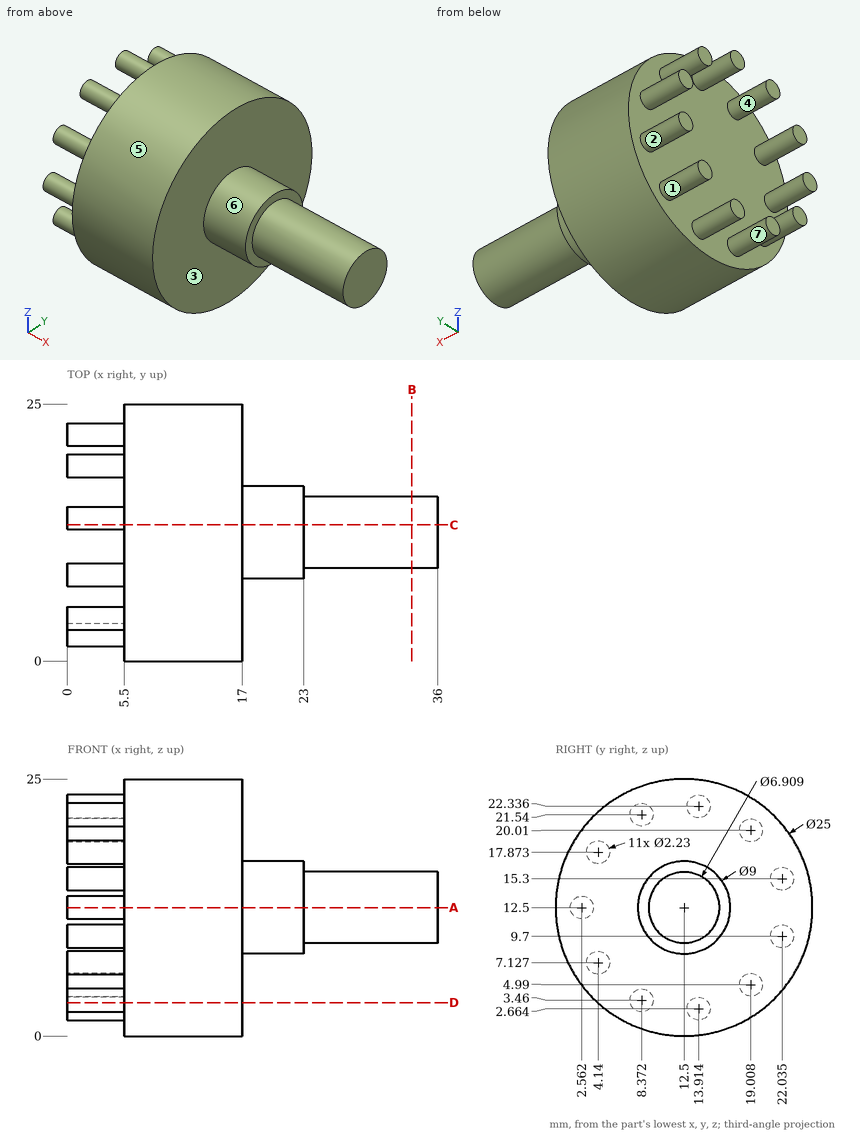
Here's the drawing with two shaded views (mm, measured from the low corner). I have some questions. A direction names the side the tool comes from. Give positions to 0.01 mm unless a question says otherwise; leave off trailing zeros. Write each loop counter-clockwise with the first axis right and the second up, starting at its lowest first coordinate (ties: lowest second). Pieces come first, ordered by that corner, then holes. Notation, with made-up numbers: (66.25, -36) -> (109.25, -36) arc R25 ccw to (109.25, -17) -> close; hole circle Ø8 at (83, 0.5). An arc over 180 degrees is marked (long way). Use one line per item in the form item = value. Start each with the question number.
1. Imagine slicing it at C-C on y = 13.25. List the corners of the cut face in (x, z) for me.
2. Imagine slicing it at A-A on z = 12.5. List the corners of the cut face in (x, y) for me (1 decimal).
3. On a 3-axis mill with a long thin cutter (end or side, diameter ignored), from which of +Z, -Z, +X, -X, +Y, -Y can I reach the whole of each face in a straight line? I mean the marked faces 5, 6 and 7. Say none if no direction works.
4. Will these pins go through, and if not, where does the flat tip stop? pin 1 Ø12 at (x, z) = (11.5, 19) entering from -Y; pin 2 Ø8 at (x, z) = (4.5, 3.5) entering from -Y; pin 3 Ø2 at (x, y) = (11.5, 2.5) entering from -Z (1 decimal).
5. If I drill on L1, parallel to X at y = 16.5, z = 21.25; L2, parallel to Z at x = 3, y = 2.5; L3, parallel to X at y = 8.5, z = 2.75, over which ranges is the centre line in solid material (lowest first)?
6. Imagine slicing it at D-D on z = 3.25. List the corners of the cut face in (x, y) for me.
7. Thinking about a two-plate mould opening in Y: for the marked faces 1, 2, 3 and 4, which applies, +Y half, -Y half, draft (parallel to the pull), parting line (faces both ways), or undercut?
8. Imagine slicing it at B-B on x = 33.5. List the corners of the cut face in (y, z) for me (1 decimal), plus the area to 3 significant figures.
Entries:
q1.outline = (0, 1.77) -> (5.5, 1.77) -> (5.5, 0.02) -> (17, 0.02) -> (17, 8.06) -> (23, 8.06) -> (23, 9.13) -> (36, 9.13) -> (36, 15.87) -> (23, 15.87) -> (23, 16.94) -> (17, 16.94) -> (17, 24.98) -> (5.5, 24.98) -> (5.5, 23.23) -> (0, 23.23) -> (0, 21.44) -> (5.5, 21.44) -> (5.5, 3.56) -> (0, 3.56) -> close
q2.outline = (0, 1.4) -> (5.5, 1.4) -> (5.5, 0) -> (17, 0) -> (17, 8) -> (23, 8) -> (23, 9) -> (36, 9) -> (36, 16) -> (23, 16) -> (23, 17) -> (17, 17) -> (17, 25) -> (5.5, 25) -> (5.5, 3.7) -> (0, 3.7) -> close
q3.face_5 = +X, -X
q3.face_6 = +X
q3.face_7 = -X
q4.pin_1 = 0.01
q4.pin_2 = 1.1
q4.pin_3 = 3.8
q5.L1 = 5.5 to 17
q5.L2 = 11.39 to 13.61
q5.L3 = 0 to 17
q6.outline = (0, 7.28) -> (5.5, 7.28) -> (5.5, 4.09) -> (17, 4.09) -> (17, 20.91) -> (5.5, 20.91) -> (5.5, 14.86) -> (0, 14.86) -> (0, 12.97) -> (5.5, 12.97) -> (5.5, 9.47) -> (0, 9.47) -> close
q7.face_1 = undercut
q7.face_2 = parting line
q7.face_3 = draft
q7.face_4 = undercut
q8.outline = circle Ø6.9 at (12.5, 12.5)
q8.area = 37.5 mm²
